```python
from build123d import *

# Parameters (mm, degrees)
BOSS_EXTRUDE1_DEPTH = 203.2
CAVITY1_START       = -39.91
CAVITY1_DEPTH       = 23.46
CAVITY1_START_2     = -18.031
CAVITY1_2_OUTLINE_W = 6.885
CAVITY1_2_OUTLINE_H = 2.04
CAVITY1_2_OUTLINE_R = 14.28
CAVITY1_2_DEPTH     = 3.581
CAVITY1_START_3     = -19.612
CAVITY1_3_DEPTH     = 3.162
CAVITY1_START_4     = 132.705
CAVITY1_4_OUTLINE_R = 2.1675
CAVITY1_4_DEPTH     = 32.64
CAVITY1_START_5     = 163.305
CAVITY1_5_DEPTH     = 2.04
CAVITY1_6_OUTLINE_R = 2.1675
CAVITY1_6_DEPTH     = 19.992
CAVITY1_7_OUTLINE_R = 2.1675
CAVITY1_7_DEPTH     = 19.992
CUT_EXTRUDE1_DEPTH  = 210.058488467
CUT_EXTRUDE2_DEPTH  = 209.983650662
SKETCH4_W           = 4.335
SKETCH4_H           = 30.6
CUT_EXTRUDE3_DEPTH  = 209.062749189
CUT_EXTRUDE4_DEPTH  = 132.705
CUT_EXTRUDE5_DEPTH  = 15
CUT_EXTRUDE6_DEPTH  = 6
CUT_EXTRUDE7_REACH  = 84.598
SKETCH8_W           = 7
SKETCH8_H           = 5
BOSS_EXTRUDE2_DEPTH = 10
CUT_EXTRUDE8_DEPTH  = 15


with BuildPart() as part:
    # Sketch1 → Boss-Extrude1 (new body)
    with BuildSketch(Plane.XY):
        with BuildLine():
            Line((42.035699114, -14.45), (-42.035699114, -14.45))
            ThreePointArc((-42.035699114, -14.45), (0, -44.45), (42.035699114, -14.45))
        make_face()
    extrude(amount=BOSS_EXTRUDE1_DEPTH)

    # Cavity1: read off the stored shape, not the designer's step
    # Cavity1 outline → Cavity1 (cut)
    with BuildSketch(Plane(origin=(0, 0, 0), x_dir=(1, 0, 0), z_dir=(0, 1, 0)).offset(CAVITY1_START)):
        with BuildLine():
            Line((16.065, -165.345), (16.065, -163.305))
            Line((16.065, -163.305), (-16.065, -163.305))
            Line((-16.065, -163.305), (-16.065, -165.345))
            Line((-16.065, -165.345), (-16.065, -183.45))
            ThreePointArc((-16.065, -183.45), (0, -199.515), (16.065, -183.45))
            Line((16.065, -183.45), (16.065, -165.345))
        make_face()
    extrude(amount=CAVITY1_DEPTH, mode=Mode.SUBTRACT)

    # Cavity1 2 outline → Cavity1 2 (cut)
    with BuildSketch(Plane(origin=(0, 0, 0), x_dir=(1, 0, 0), z_dir=(0, 1, 0)).offset(CAVITY1_START_2)):
        with Locations((19.5075, -164.325)):
            Rectangle(CAVITY1_2_OUTLINE_W, CAVITY1_2_OUTLINE_H)
        with Locations((-19.5075, -164.325)):
            Rectangle(CAVITY1_2_OUTLINE_W, CAVITY1_2_OUTLINE_H)
        with Locations((0, -183.45)):
            Circle(CAVITY1_2_OUTLINE_R)
    extrude(amount=CAVITY1_2_DEPTH, mode=Mode.SUBTRACT)

    # Cavity1 3 outline → Cavity1 3 (cut)
    with BuildSketch(Plane(origin=(0, 0, 0), x_dir=(1, 0, 0), z_dir=(0, 1, 0)).offset(CAVITY1_START_3)):
        with BuildLine():
            Line((19.89, -163.305), (16.065, -163.305))
            Line((16.065, -163.305), (16.065, -183.45))
            ThreePointArc((16.065, -183.45), (0, -199.515), (-16.065, -183.45))
            Line((-16.065, -183.45), (-16.065, -163.305))
            Line((-16.065, -163.305), (-19.89, -163.305))
            Line((-19.89, -163.305), (-19.89, -191.865))
            Line((-19.89, -191.865), (-8.555, -203.2))
            Line((-8.555, -203.2), (8.555, -203.2))
            Line((8.555, -203.2), (19.89, -191.865))
            Line((19.89, -191.865), (19.89, -163.305))
        make_face()
    extrude(amount=CAVITY1_3_DEPTH, mode=Mode.SUBTRACT)

    # Cavity1 4 outline → Cavity1 4 (cut)
    with BuildSketch(Plane.XY.offset(CAVITY1_START_4)):
        with Locations((8.925, -29.71)):
            Circle(CAVITY1_4_OUTLINE_R)
        with Locations((-8.925, -29.71)):
            Circle(CAVITY1_4_OUTLINE_R)
    extrude(amount=CAVITY1_4_DEPTH, mode=Mode.SUBTRACT)

    # Cavity1 5 outline → Cavity1 5 (cut)
    with BuildSketch(Plane.XY.offset(CAVITY1_START_5)):
        Polygon((9.131481481, -14.45), (7.65, -16.45), (16.065, -16.45), (16.065, -14.45), align=None)
        Polygon((-16.065, -16.45), (-7.65, -16.45), (-9.131481481, -14.45), (-16.065, -14.45), align=None)
    extrude(amount=CAVITY1_5_DEPTH, mode=Mode.SUBTRACT)


with BuildPart() as body_2:
    # Cavity1 6 outline → Cavity1 6 (new body)
    with BuildSketch(Plane.XY.offset(CAVITY1_START_5)):
        with Locations((-8.925, -29.71)):
            Circle(CAVITY1_6_OUTLINE_R)
    extrude(amount=CAVITY1_6_DEPTH)


with BuildPart() as body_3:
    # Cavity1 7 outline → Cavity1 7 (new body)
    with BuildSketch(Plane.XY.offset(CAVITY1_START_5)):
        with Locations((8.925, -29.71)):
            Circle(CAVITY1_7_OUTLINE_R)
    extrude(amount=CAVITY1_7_DEPTH)


with BuildPart() as cut_extrude1_tool:
    # Sketch2 → Cut-Extrude1 (new, through all)
    with BuildSketch(Plane(origin=(0, -39.91, 0), x_dir=(1, 0, 0), z_dir=(0, 1, 0))):
        with BuildLine():
            Line((16.065, -183.45), (16.065, -163.305))
            Line((16.065, -163.305), (-16.065, -163.305))
            Line((-16.065, -163.305), (-16.065, -183.45))
            ThreePointArc((-16.065, -183.45), (0, -199.515), (16.065, -183.45))
        make_face()
    extrude(amount=CUT_EXTRUDE1_DEPTH)


with BuildPart() as part_1:
    add(part.part)

    # Cut-Extrude1: cut by cut_extrude1_tool
    add(cut_extrude1_tool.part, mode=Mode.SUBTRACT)

    # Sketch3 → Cut-Extrude2 (cut, through all)
    with BuildSketch(Plane(origin=(0, -19.612, 0), x_dir=(1, 0, 0), z_dir=(0, 1, 0))):
        with BuildLine():
            Line((-8.555, -203.2), (8.555, -203.2))
            Line((8.555, -203.2), (19.89, -191.865))
            Line((19.89, -191.865), (19.89, -163.305))
            Line((19.89, -163.305), (16.065, -163.305))
            Line((16.065, -163.305), (16.065, -183.45))
            ThreePointArc((16.065, -183.45), (0, -199.515), (-16.065, -183.45))
            Line((-16.065, -183.45), (-16.065, -163.305))
            Line((-16.065, -163.305), (-19.89, -163.305))
            Line((-19.89, -163.305), (-19.89, -191.865))
            Line((-19.89, -191.865), (-8.555, -203.2))
        make_face()
    extrude(amount=CUT_EXTRUDE2_DEPTH, mode=Mode.SUBTRACT)

    # Sketch4 → Cut-Extrude3 (cut, through all)
    with BuildSketch(Plane(origin=(0, -29.71, 0), x_dir=(1, 0, 0), z_dir=(0, 1, 0))):
        with Locations((-8.925, -148.005)):
            Rectangle(SKETCH4_W, SKETCH4_H)
        with Locations((8.925, -148.005)):
            Rectangle(SKETCH4_W, SKETCH4_H)
    extrude(amount=CUT_EXTRUDE3_DEPTH, mode=Mode.SUBTRACT)

    # Sketch1<3> → Cut-Extrude4 (cut)
    with BuildSketch(Plane.XY):
        with BuildLine():
            ThreePointArc((44.45, 0), (-7.325151001, 43.842270274), (-42.035699114, -14.45))
            Line((-42.035699114, -14.45), (42.035699114, -14.45))
            ThreePointArc((42.035699114, -14.45), (43.842270274, -7.325151001), (44.45, 0))
        make_face()
        with BuildLine():
            Line((42.035699114, -14.45), (-42.035699114, -14.45))
            ThreePointArc((-42.035699114, -14.45), (0, -44.45), (42.035699114, -14.45))
        make_face()
    extrude(amount=CUT_EXTRUDE4_DEPTH, mode=Mode.SUBTRACT)

    # Sketch5 → Cut-Extrude5 (cut)
    with BuildSketch(Plane(origin=(0, 0, 132.705), x_dir=(-1, 0, 0), z_dir=(0, 0, -1))):
        with BuildLine():
            Line((6.7575, -29.71), (6.7575, -14.45))
            Line((6.7575, -14.45), (-6.7575, -14.45))
            Line((-6.7575, -14.45), (-6.7575, -29.71))
            ThreePointArc((-6.7575, -29.71), (-8.925, -31.8775), (-11.0925, -29.71))
            Line((-11.0925, -29.71), (-11.0925, -14.45))
            Line((-11.0925, -14.45), (-42.035699114, -14.45))
            ThreePointArc((-42.035699114, -14.45), (0, -44.45), (42.035699114, -14.45))
            Line((42.035699114, -14.45), (11.0925, -14.45))
            Line((11.0925, -14.45), (11.0925, -29.71))
            ThreePointArc((11.0925, -29.71), (8.925, -31.8775), (6.7575, -29.71))
        make_face()
    extrude(amount=-CUT_EXTRUDE5_DEPTH, mode=Mode.SUBTRACT)

    # Sketch6 → Cut-Extrude6 (cut, symmetric)
    with BuildSketch(Plane(origin=(0, -19.612, 0), x_dir=(1, 0, 0), z_dir=(0, 1, 0))):
        with BuildLine():
            Line((-16.065, -163.305), (-22.95, -163.305))
            Line((-22.95, -163.305), (-22.95, -165.345))
            Line((-22.95, -165.345), (-19.89, -165.345))
            Line((-19.89, -165.345), (-19.89, -191.865))
            Line((-19.89, -191.865), (-8.555, -203.2))
            Line((-8.555, -203.2), (8.555, -203.2))
            Line((8.555, -203.2), (19.89, -191.865))
            Line((19.89, -191.865), (19.89, -165.345))
            Line((19.89, -165.345), (22.95, -165.345))
            Line((22.95, -165.345), (22.95, -163.305))
            Line((22.95, -163.305), (16.065, -163.305))
            Line((16.065, -163.305), (16.065, -183.45))
            ThreePointArc((16.065, -183.45), (0, -199.515), (-16.065, -183.45))
            Line((-16.065, -183.45), (-16.065, -163.305))
        make_face()
    extrude(amount=CUT_EXTRUDE6_DEPTH, both=True, mode=Mode.SUBTRACT)

    # Sketch7 → Cut-Extrude7 (cut, up to next)
    with BuildSketch(Plane(origin=(0, 0, 147.705), x_dir=(-1, 0, 0), z_dir=(0, 0, -1)), mode=Mode.PRIVATE) as cut_extrude7_sk1:
        with BuildLine():
            Line((-11.0925, -29.71), (-11.0925, -34.71))
            ThreePointArc((-11.0925, -34.71), (-8.925, -36.8775), (-6.7575, -34.71))
            Line((-6.7575, -34.71), (-6.7575, -29.71))
            Line((-6.7575, -29.71), (-11.0925, -29.71))
        make_face()
    cut_extrude7_tool1 = extrude(cut_extrude7_sk1.sketch, amount=-CUT_EXTRUDE7_REACH, mode=Mode.PRIVATE) & part_1.part
    # Sketch7 → Cut-Extrude7 (cut, up to next)
    with BuildSketch(Plane(origin=(0, 0, 147.705), x_dir=(-1, 0, 0), z_dir=(0, 0, -1)), mode=Mode.PRIVATE) as cut_extrude7_sk2:
        with BuildLine():
            Line((11.0925, -29.71), (11.0925, -34.71))
            ThreePointArc((11.0925, -34.71), (8.925, -36.8775), (6.7575, -34.71))
            Line((6.7575, -34.71), (6.7575, -29.71))
            Line((6.7575, -29.71), (11.0925, -29.71))
        make_face()
    cut_extrude7_tool2 = extrude(cut_extrude7_sk2.sketch, amount=-CUT_EXTRUDE7_REACH, mode=Mode.PRIVATE) & part_1.part
    add(cut_extrude7_tool1.solids().sort_by_distance((8.925, -33.078635, 147.705))[0], mode=Mode.SUBTRACT)
    add(cut_extrude7_tool2.solids().sort_by_distance((-8.925, -33.078635, 147.705))[0], mode=Mode.SUBTRACT)

    # Sketch8 → Boss-Extrude2 (add)
    with BuildSketch(Plane(origin=(0, -14.45, 0), x_dir=(1, 0, 0), z_dir=(0, 1, 0))):
        with Locations((-19.45, -160.805)):
            Rectangle(SKETCH8_W, SKETCH8_H)
        with Locations((19.45, -160.805)):
            Rectangle(SKETCH8_W, SKETCH8_H)
    extrude(amount=BOSS_EXTRUDE2_DEPTH)

    # Sketch9 → Cut-Extrude8 (cut)
    with BuildSketch(Plane(origin=(0, 0, 147.705), x_dir=(-1, 0, 0), z_dir=(0, 0, -1))):
        with BuildLine():
            Line((-12, -39.799561914), (-12, -42.799561914))
            ThreePointArc((-12, -42.799561914), (0, -44.45), (12, -42.799561914))
            Line((12, -42.799561914), (12, -39.799561914))
            Line((12, -39.799561914), (16, -39.799561914))
            Line((16, -39.799561914), (16, -37.799561914))
            Line((16, -37.799561914), (-16, -37.799561914))
            Line((-16, -37.799561914), (-16, -39.799561914))
            Line((-16, -39.799561914), (-12, -39.799561914))
        make_face()
    extrude(amount=-CUT_EXTRUDE8_DEPTH, mode=Mode.SUBTRACT)


with BuildPart() as body_2_1:
    add(body_2.part)

    # Cut-Extrude1: cut by cut_extrude1_tool
    add(cut_extrude1_tool.part, mode=Mode.SUBTRACT)


with BuildPart() as body_3_1:
    add(body_3.part)

    # Cut-Extrude1: cut by cut_extrude1_tool
    add(cut_extrude1_tool.part, mode=Mode.SUBTRACT)


solid = part_1.part
```
Check sheet for the modelled part. Datum: model origin and axes. Units: mm. A direction names the side the tool comes from. Round coordinates to 2 decimals unless told otherwise and drop trailing zeros. Order: outer loops, then holes, each group sorted by start corner. A loop starts at its lowest first (then second) coordinate and runs counter-clockwise, first axis right, second up. Notation, with made-up numbers: (50.25, -4) - (109.25, -4) arc R16 cw to (109.25, 18) - close; hole circle Ø11 at (39, 35). An arc over 180 degrees is marked (long way). Answer as CSV lines item,"result". Start each with the question number.
1) Scan lines: probe 1 along X at (y, z) = (-9.5, 159); probe 2 along Y at (x, z) = (14.5, 157.5); probe 3 along Z at (x, y) = (-19, -7.5) (3 decimals). Record each from-to range of solid material in increasing order.
2) Section check B-B (x = 0). Record the cut outline in (y, z) (3 decimals).
3) Section check C-C (z = 169). Record the cut outline in (x, y) (3 decimals).
4) Section check A-A (y = -6.5). Record the cut outline in (x, z) (3 decimals), then the cut area to 3 significant figures.
5) Draft check along Z on faces 5 (the face through (-1, -26, 203.2)), 6 (the face through (-0.35, -32.86, 199.51)), 7 (the face through (29, -14.45, 175)). Enter one of: +Z half, -Z half, draft (parallel to the pull), parting line (faces both ways), or undercut.
6) Tool access check on faces 1 (the face through (6.758, -25, 155)), 2 (the face through (0, -37.8, 155)), 3 (the face through (0, -39.91, 181)), 4 (the face through (12, -41, 155)). Record the directions out of +Z, -Z, +X, -X, +Y, -Y that give a thin tool (end or side, any length) a straight path to the whole face; none if there is none.
7) Depth check by flat-ended pin: pin 1 (5.5 mm diameter, centred on y = -10.5, z = 161.5, fed in from -X); pin 2 (1.2 mm diameter, centred on x = 14.5, z = 154, fed in from +Y); pin 3 (5 mm diameter, centred on y = -26, z = 194.5, fed in from -X); pin 4 (7.5 mm diameter, centred on x = -5, y = -40.5, fed in from -Z) (3 decimals). Enter the tip coordinate at first touch or a pass-through.
8) Section check D-D (y = -21.5). Give the number of separate pieces and of enclosed holes in the cut face, then the cut area to 3 significant figures.
Determined:
1,probe 1,"-22.95 to -15.95, 15.95 to 22.95"
1,probe 2,"-42.02 to -39.8, -37.8 to -14.45"
1,probe 3,"158.305 to 163.305"
2,outline,"(-44.45, 162.705) - (-37.8, 162.705) - (-37.8, 147.705) - (-14.45, 147.705) - (-14.45, 163.305) - (-39.91, 163.305) - (-39.91, 199.515) - (-25.612, 199.515) - (-25.612, 203.2) - (-44.45, 203.2) - close"
3,outline,"(-42.036, -14.45) arc R44.45 ccw to (42.036, -14.45) - (19.89, -14.45) - (19.89, -25.612) - (16.065, -25.612) - (16.065, -39.91) - (-16.065, -39.91) - (-16.065, -25.612) - (-19.89, -25.612) - (-19.89, -14.45) - close"
4,outline,"(-22.95, 158.305) - (-15.95, 158.305) - (-15.95, 163.305) - (-22.95, 163.305) - close; (15.95, 158.305) - (22.95, 158.305) - (22.95, 163.305) - (15.95, 163.305) - close"
4,area,"70.0 mm^2"
5,face 5,"+Z half"
5,face 6,"undercut"
5,face 7,"draft"
6,face 1,"-Z, +Y"
6,face 2,"-Z"
6,face 3,"+Y"
6,face 4,"-Z, -Y"
7,pin 1,"x = -22.95"
7,pin 2,"y = -14.45"
7,pin 3,"x = -37.73"
7,pin 4,"z = 147.705"
8,separate pieces,"3"
8,enclosed holes,"0"
8,area,"2,710 mm^2"
